The model under review builds one solid part; all positions refer to its coordinate system, in mm. Face numbers are marked on the shaded views. A direction names the side the tool comes from. Round coordinates to 2 decimals unless told otherwise and drop trailing zeros. Write each loop counter-clockwise with the first axis right and the second up, starting at its lowest first coordinate (ties: lowest second). Pieces come first, ordered by that corner, then holes. Notation, with made-up numbers: (-39, -23.75) - (16, -23.75) arc R20 ccw to (16, 13.25) - close; hole circle Ø5 at (9, 42). An arc over 180 degrees is marked (long way). Use one line per item in the form item = value.
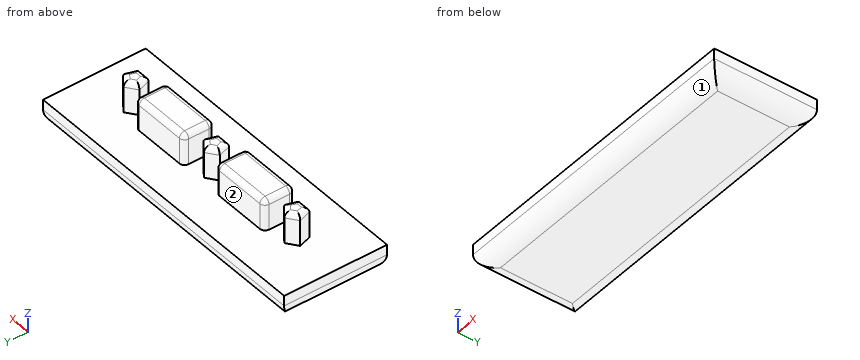
from build123d import *

# Parameters (mm, degrees)
F0_W     = 60
F0_H     = 20
F2_DEPTH = 5
F1_W     = 12
F1_H     = 6
F3_DEPTH = 6
F4_R     = 3
F5_R     = 1


with BuildPart() as f2:
    # F0 (on Top) → F2 (new body)
    with BuildSketch(Plane.XY):
        with Locations((30, 10)):
            Rectangle(F0_W, F0_H)
    extrude(amount=-F2_DEPTH)

    # F1 (on face) → F3 (join)
    with BuildSketch(Plane.XY):
        Polygon((8.736262, 8.260613), (11.263738, 8.260613), (12.044772, 10.664387), (10, 12.15), (7.955228, 10.664387), align=None)
        Polygon((30, 12.15), (27.955228, 10.664387), (28.736262, 8.260613), (31.263738, 8.260613), (32.044772, 10.664387), align=None)
        Polygon((50, 12.15), (47.955228, 10.664387), (48.736262, 8.260613), (51.263738, 8.260613), (52.044772, 10.664387), align=None)
        with Locations((20, 10)):
            Rectangle(F1_W, F1_H)
        with Locations((40, 10)):
            Rectangle(F1_W, F1_H)
    extrude(amount=F3_DEPTH)

    # F4
    f4_edges = [f2.edges().sort_by_distance(p)[0] for p in [
        (0, 10, -5),
        (30, 0, -5),
        (60, 10, -5),
        (30, 20, -5),
    ]]
    fillet(f4_edges, radius=F4_R)

    # F5
    f5_edges = [f2.edges().sort_by_distance(p)[0] for p in [
        (8.977614, 11.407193, 6),
        (8.345745, 9.4625, 6),
        (10, 8.260613, 6),
        (11.654255, 9.4625, 6),
        (11.022386, 11.407193, 6),
        (28.977614, 11.407193, 6),
        (28.345745, 9.4625, 6),
        (30, 8.260613, 6),
        (31.654255, 9.4625, 6),
        (31.022386, 11.407193, 6),
        (51.654255, 9.4625, 6),
        (50, 8.260613, 6),
        (48.345745, 9.4625, 6),
        (48.977614, 11.407193, 6),
        (51.022386, 11.407193, 6),
        (14, 7, 3),
        (26, 7, 3),
        (26, 13, 3),
        (14, 13, 3),
        (34, 13, 3),
        (34, 7, 3),
        (46, 13, 3),
        (46, 7, 3),
        (14, 10, 6),
        (20, 13, 6),
        (26, 10, 6),
        (20, 7, 6),
        (34, 10, 6),
        (40, 13, 6),
        (46, 10, 6),
        (40, 7, 6),
    ]]
    fillet(f5_edges, radius=F5_R)


solid = f2.part
(1) Add section A-A on z = 1.75. Count the separate pieces of the cut face and the enclosed holes in it, then the cut area to 3 significant figures.
Geometry results:
separate_pieces = 5
enclosed_holes = 0
area = 175 mm2
(2) Insertion check: P1, Ø3, axis at x = 10, z = 2, coming from the -Y side; P2, Ø6, axis at x = 37, z = 4, coming from the +Y side; P3, Ø1.5, axis at x = 38, z = 2.5, coming from the -Y side. Each pin has a flat end and moves straight along its axis. Give the tip position at first contact, or say it passes through.
Geometry results:
P1 = 8.26
P2 = 13
P3 = 7
(3) Machinability: for the marked faces 1 and 2, which of the approach directions +Z, -Z, +X, -X, +Y, -Y give a long, thin tool a straight path to every point of the face, cutting with its end or side? Answer none if there is none.
Geometry results:
face_1 = -Z, +X, -X, -Y
face_2 = +Z, +X, -X, +Y
(4) Add section C-C on y = 14.75. Write out the cut boundary in (x, z).
Geometry results:
outline = (0, -2) arc R3 ccw to (3, -5) - (57, -5) arc R3 ccw to (60, -2) - (60, 0) - (0, 0) - close
(5) To check wall thickness, follow L1, parallel to X at y = 8.75, z = 3.5; L2, parallel to X at y = 9.25, z = 2.25; L3, parallel to Y at x = 18.5, z = -2.25. State the ranges of each line that lie inside material, in increasing order.
Geometry results:
L1 = 8.58 to 11.42, 14 to 26, 28.58 to 31.42, 34 to 46, 48.58 to 51.42
L2 = 8.41 to 11.59, 14 to 26, 28.41 to 31.59, 34 to 46, 48.41 to 51.59
L3 = 0.01 to 19.99
(6) Add section D-D on z = -3. Write out the cut boundary in (x, y), then the cut area to 3 significant figures.
Geometry results:
outline = (0.17, 0.17) - (59.83, 0.17) - (59.83, 19.83) - (0.17, 19.83) - close
area = 1,170 mm2
(7) Add section B-B on x = 21.5. Write out the cut boundary in (y, z), then the cut area to 3 significant figures.
Geometry results:
outline = (0, -2) arc R3 ccw to (3, -5) - (17, -5) arc R3 ccw to (20, -2) - (20, 0) - (13, 0) - (13, 5) arc R1 ccw to (12, 6) - (8, 6) arc R1 ccw to (7, 5) - (7, 0) - (0, 0) - close
area = 132 mm2
